CAD build for the part. Positions are in the model's coordinates, mm. Face numbers are marked on the shaded views. A direction names the side the tool comes from. Round coordinates to 2 decimals unless told otherwise and drop trailing zeros. Loops run counter-clockwise (first coordinate to the right, second up) from the corner with the lowest first, then second, coordinate; pieces in that order, holes last. Notation, with made-up numbers: M -14.75,82 L 19.25,82 A11 cw 19.25,92 Z; hole C 8,-19 d1. An arc over 180 degrees is marked long. Use one line per item in the form item = value.
from build123d import *

# Parameters (mm, degrees)
F1_DEPTH = 76.2
F2_W     = 28.575
F2_H     = 34.19415
F3_DEPTH = 33.782
F4_R     = 4.699
F5_DEPTH = 53.594


with BuildPart() as f1:
    # F0 (on Right) → F1 (new body)
    with BuildSketch(Plane.YZ):
        Polygon((-28.850567, 0), (-28.850567, -19.05), (66.399433, -19.05), (66.399433, 0), (40.999433, 0), (40.999433, 50.8), (15.599433, 50.8), (15.599433, 0), align=None)
    extrude(amount=F1_DEPTH)

    # F2 (on face) → F3 (cut)
    with BuildSketch(Plane.XZ.offset(-15.599433)):
        with Locations((39.112404, 33.702925)):
            Rectangle(F2_W, F2_H)
    extrude(amount=-F3_DEPTH, mode=Mode.SUBTRACT)

    # F4 (on face) → F5 (cut)
    with BuildSketch(Plane.XY):
        with Locations((12.373271, 54.11797)):
            Circle(F4_R)
        with Locations((65.402929, 54.126016)):
            Circle(F4_R)
        with Locations((12.459423, -16.466378)):
            Circle(F4_R)
        with Locations((64.811589, -16.606646)):
            Circle(F4_R)
    extrude(amount=-F5_DEPTH, mode=Mode.SUBTRACT)


solid = f1.part
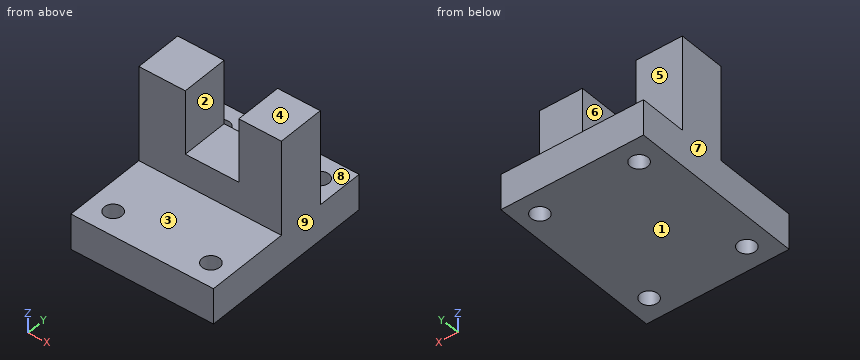
1. Probe line 1 along X through (y, z) = (57, -15); line 2 along Z through (x, y) = (10, -2); line 3 along X through (y, z) = (35, 48.5). List the from-to ranges inside material, lowest first. Write a range as from..to.
Completed:
line_1 = 0..8.66, 16.08..61.69, 69.12..76.2
line_2 = -19.05..0
line_3 = 0..24.82, 53.4..76.2
2. Cut at D-D on y = 57. Write the cut outline in (x, z).
Completed:
outline = M 0,-19.05 L 8.66,-19.05 L 8.66,0 L 0,0 Z; M 16.08,-19.05 L 61.69,-19.05 L 61.69,0 L 16.08,0 Z; M 69.12,-19.05 L 76.2,-19.05 L 76.2,0 L 69.12,0 Z
3. Drop flat-ended pins along their axis: P1, Ø3, axis at x = 63, z = 22.5, coming from the +Y side; P2, Ø6, axis at x = 60, y = 54.5, coming from the +Z side; P3, Ø15, axis at x = 31, z = 29, coming from the -Y side. Give the stop position or say it passes through.
Completed:
P1 = 41
P2 = 0
P3 = 15.6
4. Pull direction X, two halves, no side cores. Call the marked faces 6, 7, 8 and 9: +X half, -X half, draft (parallel to the pull), parting line (faces both ways), or undercut.
Completed:
face_6 = undercut
face_7 = -X half
face_8 = draft
face_9 = +X half
5. Cut at B-B on y = 34. Write the cut outline in (x, z), and give its area (3 significant figures).
Completed:
outline = M 0,-19.05 L 76.2,-19.05 L 76.2,50.8 L 53.4,50.8 L 53.4,16.61 L 24.82,16.61 L 24.82,50.8 L 0,50.8 Z
area = 4,350 mm2
6. Tool access for the marked faces 1, 2, 3, 4 and 5: list every direction of +Z, -Z, +X, -X, +Y, -Y with a clear straight run to the whole face (end or side of a thin tool).
Completed:
face_1 = -Z, +X, -X, +Y, -Y
face_2 = +Z, +Y, -Y
face_3 = +Z, +X, -X, -Y
face_4 = +Z, +X, -X, +Y, -Y
face_5 = +Z, +X, -X, +Y
7. Cut at C-C on x = 44. Write the cut outline in (y, z).
Completed:
outline = M -28.85,-19.05 L 66.4,-19.05 L 66.4,0 L 41,0 L 41,16.61 L 15.6,16.61 L 15.6,0 L -28.85,0 Z
8. Cut at A-A on z = 45. Write the cut outline in (x, y).
Completed:
outline = M 0,15.6 L 24.82,15.6 L 24.82,41 L 0,41 Z; M 53.4,15.6 L 76.2,15.6 L 76.2,41 L 53.4,41 Z
